Could you check a few things on this model? Use its own coordinates, in mm. Face numbers are marked on the shaded views. A direction names the side the tool comes from. Give positions to 0.01 mm unless a question says otherwise; leave off trailing zeros. Loops run counter-clockwise (first coordinate to the right, second up) from the corner with the lowest first, then second, coordinate; pieces in that order, holes last.
1. For the marked faces 4, 5 and 6, which set-ups out of +Z, -Z, +X, -X, +Y, -Y let a thin tool reach every point of the face, with its end or its side?
2. For P1, Ø8, axis at x = 11, z = 19.5, coming from the -Y side; P2, Ø18, axis at x = 8, z = 13.5, coming from the -Y side; P3, Ø19.5, axis at x = -12.5, z = -11.5, coming from the +Y side, each with a flat end and sliding along its axis, tell me the tip position at first contact or that it passes through.
3. Imagine slicing it at A-A (y = 12). List the corners of the cut face in (x, z) for me, plus the area to 3 significant figures.
4. Thinking about a two-plate mould opening in X: for the marked faces 1, 2 and 3, which applies, +X half, -X half, draft (parallel to the pull), parting line (faces both ways), or undercut?
5. Imagine slicing it at D-D (y = 53.5). List the corners of the cut face in (x, z) for me.
6. I need wall thicknesses on line 1 along X through (y, z) = (18, 0); line 2 along X through (y, z) = (43.3, 0); line 3 along Z through (x, y) = (-26.5, 58.5). Which ranges of each line are inside material? Lowest first, please.
```python
from build123d import *

# Parameters (mm, degrees)
SKETCH1_W           = 100
SKETCH1_H           = 80
SKETCH1_R           = 26
BOSS_EXTRUDE1_DEPTH = 70
SKETCH2_R           = 32.5
CUT_EXTRUDE1_DEPTH  = 27
BOSS_EXTRUDE2_START = 1
SKETCH4_R           = 32.5
SKETCH4_R_2         = 30.25
BOSS_EXTRUDE2_DEPTH = 1
SKETCH5_R           = 35
CUT_EXTRUDE2_DEPTH  = 19
CUT_EXTRUDE3_START  = -8
SKETCH6_R           = 32.5
CUT_EXTRUDE3_DEPTH  = 8
CUT_EXTRUDE4_START  = -1
SKETCH7_R           = 30.25
CUT_EXTRUDE4_DEPTH  = 1
CUT_EXTRUDE5_DEPTH  = 11


with BuildPart() as part:
    # Sketch1 → Boss-Extrude1 (new body)
    with BuildSketch(Plane(origin=(0, 0, 0), x_dir=(1, 0, 0), z_dir=(0, 1, 0))):
        Rectangle(SKETCH1_W, SKETCH1_H)
        with Locations(Location((0, 0, 0), (0, 0, 270))):
            Circle(SKETCH1_R, mode=Mode.SUBTRACT)
    extrude(amount=BOSS_EXTRUDE1_DEPTH)

    # Sketch2 → Cut-Extrude1 (cut)
    with BuildSketch(Plane(origin=(0, 70, 0), x_dir=(1, 0, 0), z_dir=(0, 1, 0))):
        with Locations(Location((0, 0, 0), (0, 0, 270))):
            Circle(SKETCH2_R)
    extrude(amount=-CUT_EXTRUDE1_DEPTH, mode=Mode.SUBTRACT)

    # Sketch4 → Boss-Extrude2 (add)
    with BuildSketch(Plane(origin=(0, 43, 0), x_dir=(1, 0, 0), z_dir=(0, 1, 0)).offset(BOSS_EXTRUDE2_START)):
        with Locations(Location((0, 0, 0), (0, 0, 270))):
            Circle(SKETCH4_R)
        with Locations(Location((0, 0, 0), (0, 0, 270))):
            Circle(SKETCH4_R_2, mode=Mode.SUBTRACT)
    extrude(amount=-BOSS_EXTRUDE2_DEPTH)

    # Sketch5 → Cut-Extrude2 (cut)
    with BuildSketch(Plane(origin=(0, 70, 0), x_dir=(1, 0, 0), z_dir=(0, 1, 0))):
        with Locations(Location((0, 0, 0), (0, 0, 270))):
            Circle(SKETCH5_R)
    extrude(amount=-CUT_EXTRUDE2_DEPTH, mode=Mode.SUBTRACT)

    # Sketch6 → Cut-Extrude3 (cut)
    with BuildSketch(Plane.XZ.offset(CUT_EXTRUDE3_START)):
        with Locations(Location((0, 0, 0), (0, 0, 90))):
            Circle(SKETCH6_R)
    extrude(amount=CUT_EXTRUDE3_DEPTH, mode=Mode.SUBTRACT)

    # Sketch7 → Cut-Extrude4 (cut)
    with BuildSketch(Plane.XZ.offset(-8).offset(CUT_EXTRUDE4_START)):
        with Locations(Location((0, 0, 0), (0, 0, 90))):
            Circle(SKETCH7_R)
    extrude(amount=CUT_EXTRUDE4_DEPTH, mode=Mode.SUBTRACT)

    # Sketch8 → Cut-Extrude5 (cut)
    with BuildSketch(Plane(origin=(0, 70, 0), x_dir=(1, 0, 0), z_dir=(0, 1, 0))):
        with BuildLine():
            Line((50, 40), (0, 40))
            ThreePointArc((0, 40), (28.284271247, 28.284271247), (40, 0))
            ThreePointArc((40, 0), (28.284271247, -28.284271247), (0, -40))
            Line((0, -40), (50, -40))
            Line((50, -40), (50, 40))
        make_face()
        with BuildLine():
            Line((0, 40), (-50, 40))
            Line((-50, 40), (-50, -40))
            Line((-50, -40), (0, -40))
            ThreePointArc((0, -40), (-40, 0), (0, 40))
        make_face()
    extrude(amount=-CUT_EXTRUDE5_DEPTH, mode=Mode.SUBTRACT)


solid = part.part
```
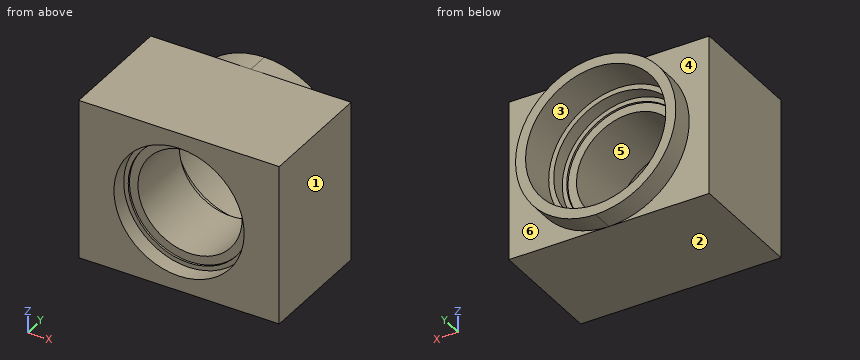
Derived:
1. face 4: -X, +Y
1. face 5: +Y, -Y
1. face 6: +X, +Y
2. P1: stops at y = 9
2. P2: passes through
2. P3: stops at y = 43
3. outline: (-50, -40) - (50, -40) - (50, 40) - (-50, 40) - close; hole circle Ø52 at (0, 0)
3. area: 5,880 mm2
4. face 1: +X half
4. face 2: draft
4. face 3: undercut
5. outline: (-50, -40) - (50, -40) - (50, 40) - (-50, 40) - close; hole circle Ø70 at (0, 0)
6. line 1: x = -50 to -26, 26 to 50
6. line 2: x = -50 to -30.25, 30.25 to 50
6. line 3: z = -40 to -22.86, 22.86 to 40
